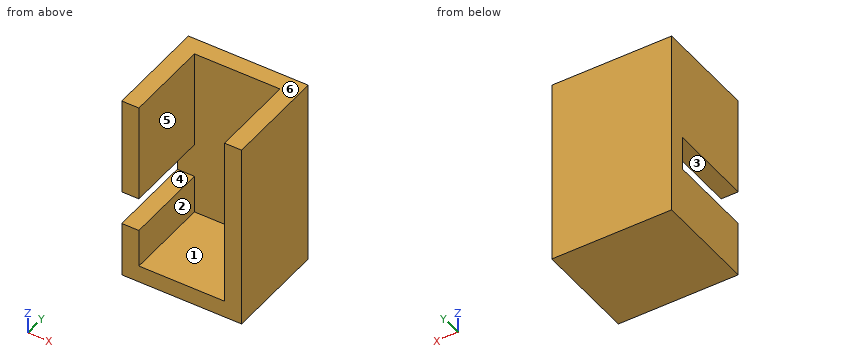
Autodesk Inventor part; units mm, degrees
ref_plane "YZ Plane" through (0, 0, 0) normal (1, 0, 0) x (0, 1, 0)
ref_plane "XZ Plane" through (0, 0, 0) normal (0, 1, 0) x (-1, 0, 0)
ref_plane "XY Plane" through (0, 0, 0) normal (0, 0, 1) x (1, 0, 0)
sketch "Sketch1" plane through (0, 0, 0) normal (0, 0, 1) x (1, 0, 0)
  line L0 (0, 0) -> (14, 0)
  line L1 (14, 0) -> (14, -12)
  line L2 (14, -12) -> (0, -12)
  line L3 (0, -12) -> (0, 0)
  dimension "d0" = 14
  dimension "d1" = 12
extrude "Extrusion1" add sketch "Sketch1" against normal blind 22
sketch "Sketch2" plane through (0, 0, 0) normal (0, 0, 1) x (1, 0, 0)
  line L0 (2, -2) -> (12, -2)
  line L1 (12, -2) -> (12, -22)
  line L2 (12, -22) -> (2, -22)
  line L3 (2, -22) -> (2, -2)
  point P0 (0, 0)
  dimension "d4" = 10
  dimension "d5" = 20
extrude "Extrusion2" cut sketch "Sketch2" against normal blind 20
sketch "Sketch8" plane through (0, -12, 0) normal (-1, 0, 0) x (0, 0, 1)
  point P0 (0, 12)
sketch "Sketch9" plane through (0, -12, 0) normal (-1, 0, 0) x (0, 0, 1)
  point P0 (0, 12)
sketch "Sketch11" plane through (0, -12, 0) normal (-1, 0, 0) x (0, 0, 1)
  point P0 (0, 12)
sketch "Sketch12" plane through (0, -12, 0) normal (-1, 0, 0) x (0, 0, 1)
  line L0 (-11.5, 10) -> (-15.5, 10)
  line L1 (-15.5, 10) -> (-15.5, -1.8066)
  line L2 (-15.5, -1.8066) -> (-11.5, -1.8066)
  line L3 (-11.5, -1.8066) -> (-11.5, 10)
  point P0 (0, 12)
  dimension "d24" = 4
extrude "Extrusion8" cut sketch "Sketch12" against normal blind 10
properties part number "housing_v04"
For this review, take the finished solid that the model builds, in its own axes (mm). Face numbers are marked on the shaded views. A direction names the side the tool comes from. Coordinates: 2 decimals unless noted, no trailing zeros. Loops run counter-clockwise (first coordinate to the right, second up) from the corner with the lowest first, then second, coordinate; pieces in that order, holes last.
1. Add section C-C, the plane x = 9.25. Give the boundary of the cut face in (y, z).
2. Mouldability with a two-part tool opening along Z and no side actions: class the marked faces 1, 2, 3 and 4 as +Z half, -Z half, draft (parallel to the pull), parting line (faces both ways), or undercut.
3. For line 1 (X direction, y = -8.25, z = -9.5); line 2 (Y direction, x = 11.5, z = -0.75); line 3 (Z direction, x = 5.5, y = -10), list the stretches that pass through material, from the lowest coordinate up.
4. Insertion check: P1, Ø4, axis at x = 4.5, z = -11, coming from the -Y side. The pin has a flat end and moves straight along its axis. Give the tip position at first contact, or say it passes through.
5. Add section A-A, the plane y = -4.75. Give the boundary of the cut face in (x, z), then the cut area to 3 significant figures.
6. For the marked faces 5 and 6, list the 3-axis set-ups (+Z, -Z, +X, -X, +Y, -Y) from which the entire face can be reached by the end or side of a thin tool; tool diameter is ignored.
7. Add section B-B, the plane z = -3.75. Give the boundary of the cut face in (x, y).
Result:
1. outline: (-12, -22) - (0, -22) - (0, 0) - (-2, 0) - (-2, -20) - (-12, -20) - close
2. face 1: +Z half
2. face 2: draft
2. face 3: undercut
2. face 4: undercut
3. line 1: x = 0 to 2, 12 to 14
3. line 2: y = -2 to 0
3. line 3: z = -22 to -20
4. P1: stops at y = -2
5. outline: (0, -22) - (14, -22) - (14, 0) - (12, 0) - (12, -20) - (2, -20) - (2, -15.5) - (0, -15.5) - close; (0, -11.5) - (2, -11.5) - (2, 0) - (0, 0) - close
5. area: 100 mm2
6. face 5: +Z, -Y
6. face 6: +Z, +X, -X, +Y, -Y
7. outline: (0, -12) - (2, -12) - (2, -2) - (12, -2) - (12, -12) - (14, -12) - (14, 0) - (0, 0) - close
